Check sheet for the drawn part. Datum: minimum x, y, z corner. Units: mm. A direction names the side the tool comes from. Give positions to 0.01 mm unless a question says otherwise; leave off trailing zeros. Order: outer loops, then holes, each group sorted by start corner. A loop starts at its lowest first (then second) coordinate and runs counter-clockwise, first axis right, second up.
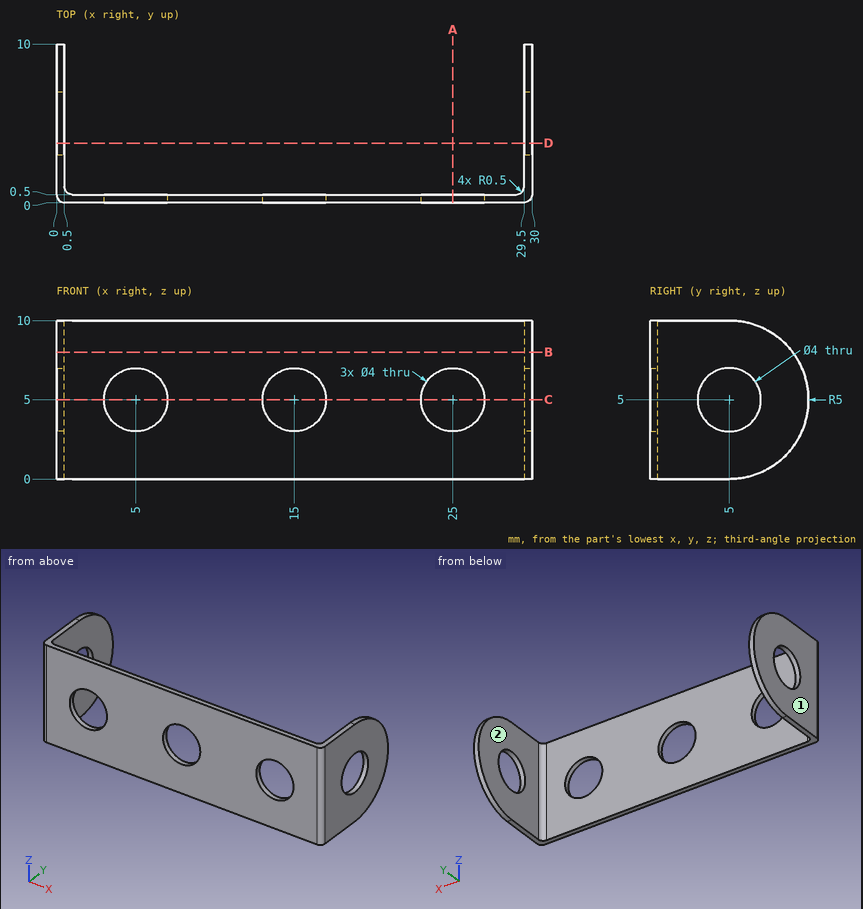
Item 1: Scan lines: L1, parallel to X at y = 5, z = 9.25; L2, parallel to X at y = 0.35, z = 5; L3, parallel to Z at x = 25, y = 0.35. Record each from-to range of solid material in increasing order.
Reported:
L1: x = 0 to 0.5, 29.5 to 30
L2: x = 0.02 to 3, 7 to 13, 17 to 23, 27 to 29.98
L3: z = 0 to 3, 7 to 10
Item 2: Sectioned sample at D-D (y = 3.75). Enter the section's corners in (x, z).
Reported:
outline: (0, 0) - (0.5, 0) - (0.5, 3.44) - (0, 3.44) - close; (0, 6.56) - (0.5, 6.56) - (0.5, 10) - (0, 10) - close; (29.5, 0) - (30, 0) - (30, 3.44) - (29.5, 3.44) - close; (29.5, 6.56) - (30, 6.56) - (30, 10) - (29.5, 10) - close
Item 3: Sectioned sample at B-B (z = 8). Enter the section's corners in (x, y), and give its area (3 significant figures).
Reported:
outline: (0, 0.5) arc R0.5 ccw to (0.5, 0) - (29.5, 0) arc R0.5 ccw to (30, 0.5) - (30, 9) - (29.5, 9) - (29.5, 1) arc R0.5 cw to (29, 0.5) - (1, 0.5) arc R0.5 cw to (0.5, 1) - (0.5, 9) - (0, 9) - close
area: 23.5 mm2
Item 4: Gauge pin test, flat ends, axial feed: pin 1 (3.5 mm diameter, centred on y = 5, z = 5, fed in from +X); pin 2 (6 mm diameter, centred on y = 4.5, z = 5, fed in from -X); pin 3 (3 mm diameter, centred on x = 9, z = 1, fed in from +Y). Record the tip position at first contact, or that the pin passes through.
Reported:
pin 1: passes through
pin 2: stops at x = 0
pin 3: stops at y = 0.5
Item 5: Set-up check for the marked faces 1 and 2: record each of +Z, -Z, +X, -X, +Y, -Y from which the full face is reachable in a straight line by a thin tool's end or side.
Reported:
face 1: +Z, -Z, -X, +Y, -Y
face 2: +Z, -Z, +Y
Item 6: Sectioned sample at A-A (x = 25). Enter the section's corners in (y, z), and give its area (3 significant figures).
Reported:
outline: (0, 0) - (0.5, 0) - (0.5, 3) - (0, 3) - close; (0, 7) - (0.5, 7) - (0.5, 10) - (0, 10) - close
area: 3.00 mm2
Item 7: Sectioned sample at C-C (z = 5). Give the number of separate pieces and of enclosed holes in the cut face, and give its area (3 significant figures).
Reported:
separate pieces: 6
enclosed holes: 0
area: 14.5 mm2
